The model under review builds one solid part; all positions refer to its coordinate system, in mm. Face numbers are marked on the shaded views. A direction names the side the tool comes from. Coordinates: 2 decimals unless noted, no trailing zeros. Loops run counter-clockwise (first coordinate to the right, second up) from the corner with the lowest first, then second, coordinate; pieces in that order, holes last. Notation, with made-up numbers: (-39, 80) -> (-18, 80) arc R13 cw to (-18, 94) -> close; hole circle Ø5 at (55.5, 72.25). An arc over 180 degrees is marked (long way). One line per question, with ' | ' between items. Start each with the question number.
from build123d import *

# Parameters (mm, degrees)
SKETCH6_W          = 28.575
SKETCH6_H          = 5.588000000000008
FILLET1_R          = 1.524
CUT_EXTRUDE1_DEPTH = 133.3733867563125


with BuildPart() as part:
    # Sweep1: sweep along a path in Sketch1
    with BuildLine(Plane(origin=(0, 0, 0), x_dir=(0, 0, -1), z_dir=(1, 0, 0))) as sweep1_path:
        Line((3.9e-16, 94.996), (0, 0))
        ThreePointArc((0, 0), (37.09799061473534, -40.48535253044856), (80.66258708241622, -7.057061940383765))
        Line((80.66258708241622, -7.057061940383765), (87.31250000000001, 30.656468291151832))
    # Sketch2 → Sweep1 (sweep)
    with BuildSketch(Plane(origin=(0, 94.996, -15.113000000000007), x_dir=(1, 0, 0), z_dir=(0, -1, 0))):
        Polygon((-12.763499999999997, 17.653000000000006), (12.763499999999997, 17.65300000000001), (12.763500000000008, 15.113000000000001), (-12.763499999999983, 15.113000000000001), align=None)
    sweep(path=sweep1_path.line)

    # Sweep3: sweep along a path in Sketch5
    with BuildLine(Plane(origin=(0, 0, 0), x_dir=(0, 0, -1), z_dir=(1, 0, 0))) as sweep3_path:
        Line((0, 63.245999999999995), (-3.47e-15, 3.35e-15))
        ThreePointArc((-3.47e-15, 3.35e-15), (37.09799061473534, -40.48535253044856), (80.66258708241622, -7.057061940383765))
        Line((80.66258708241622, -7.057061940383765), (87.31250000000001, 30.656468291151832))
    # Sketch6 → Sweep3 (sweep)
    with BuildSketch(Plane(origin=(0, 44.66337954391292, -7.875358863214053), x_dir=(1, 0, 0), z_dir=(0, 0.9848077530122094, -0.1736481776669233))):
        with Locations((7.11e-15, 81.9325870824162)):
            Rectangle(SKETCH6_W, SKETCH6_H)
        Polygon((-12.763499999999997, 83.2025870824162), (-12.763499999999983, 80.6625870824162), (12.763500000000008, 80.6625870824162), (12.763499999999997, 83.2025870824162), align=None, mode=Mode.SUBTRACT)
    sweep(path=sweep3_path.line)

    # Fillet1
    fillet1_edges = [part.edges().sort_by_distance(p)[0] for p in [
        (-14.287499999999994, 31.622999999999998, -1.5239999999999834),
        (14.287500000000007, 31.622999999999998, 4.064000000000009),
        (-14.287499999999994, -38.96715181055673, -37.23081596668276),
        (14.287500000000007, -44.53388778349341, -36.74378967620887),
        (14.287500000000009, -38.967151810556715, -37.23081596668276),
        (14.287500000000009, 31.622999999999998, -1.5240000000000133),
        (14.287500000000007, 11.09399698134567, -87.98980224944968),
        (14.287500000000009, 12.06434299814844, -82.48669652561743),
        (-14.287499999999996, -44.53388778349341, -36.74378967620887),
        (-14.287499999999996, 31.622999999999998, 4.064000000000009),
        (-14.287499999999994, 12.06434299814843, -82.48669652561752),
        (-14.287499999999996, 11.09399698134567, -87.98980224944968),
        (14.287500000000007, 30.435935105514844, -88.56320584632552),
        (5.33e-15, 29.950762097113483, -91.31475870824151),
        (-14.287499999999994, 30.435935105514847, -88.56320584632554),
        (7.11e-15, 30.92110811391625, -85.81165298440926),
    ]]
    fillet(fillet1_edges, radius=FILLET1_R)

    # Sketch9 → Cut-Extrude1 (cut, through all)
    with BuildSketch(Plane(origin=(0, 0, 0), x_dir=(-1, 0, 0), z_dir=(0, -6e-17, -1))):
        with BuildLine():
            Line((4.7625, 86.03336979368495), (4.762500000000001, 79.121))
            ThreePointArc((4.762500000000001, 79.121), (-7.9e-16, 68.57086979368498), (-4.762500000000001, 79.121))
            Line((-4.762500000000001, 79.121), (-4.7625, 86.03336979368495))
            ThreePointArc((-4.7625, 86.03336979368495), (1.48e-15, 90.79586979368496), (4.7625, 86.03336979368495))
        make_face()
    extrude(amount=-CUT_EXTRUDE1_DEPTH, mode=Mode.SUBTRACT)


solid = part.part
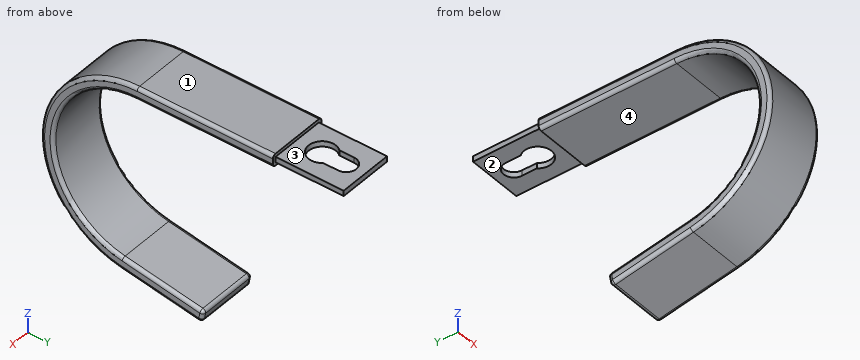
1) Consider section A-A, the plane x = 0. Write out the cut boundary in (y, z), plus the area to 3 significant figures.
2) Consider section B-B, the plane y = 72.5. Write out the cut boundary in (x, z), plus the area to 3 significant figures.
3) Machinability: for the marked faces 1, 2, 3 and 4, which of the approach directions +Z, -Z, +X, -X, +Y, -Y give a long, thin tool a straight path to every point of the face, cutting with its end or side? Answer none if there is none.
4) Consider section C-C, the plane x = 8.5. Write out the cut boundary in (y, z), plus the area to 3 significant figures.
5) Insertion check: pin 1 Ø7.5 at (x, y) = (2, 23) entering from -Z; pin 2 Ø0.8 at (y, z) = (84, 1) entering from -X; pin 3 Ø8 at (x, z) = (5.5, -27) entering from +Y. Each pin has a flat end and moves straight along its axis. Give the tip position at first contact, or say it passes through.
6) Wall thickness on L1, parallel to Z at x = 5.25, y = 69.5; L2, parallel to Z at x = 5.5, y = -26; L3, parallel to Z at x = -12.25, y = 18: over which ranges is each line inside the solid? List them lowest first.
Filled sheet:
1) outline: (-7.76, -84.66) -> (28.45, -91.05) arc R1.52 ccw to (30.22, -89.81) -> (30.66, -87.31) arc R1.52 ccw to (29.42, -85.55) -> (-6.79, -79.16) arc R39.12 cw to (0, -1.52) -> (63.25, -1.52) -> (63.25, 0) -> (68.57, 0) -> (68.57, 2.54) -> (63.25, 2.54) -> (63.25, 4.06) -> (0, 4.06) arc R44.7 ccw to start; (90.8, 0) -> (95, 0) -> (95, 2.54) -> (90.8, 2.54) -> close | area: 1,290 mm^2
2) outline: (-12.76, 0) -> (-5.87, 0) -> (-5.87, 2.54) -> (-12.76, 2.54) -> close; (5.87, 0) -> (12.76, 0) -> (12.76, 2.54) -> (5.87, 2.54) -> close | area: 35.0 mm^2
3) face 1: +Z, +X, -X, +Y, -Y | face 2: -Z, +X, -X, +Y | face 3: +Z, +X, -X, +Y | face 4: +X, -X, +Y
4) outline: (-7.76, -84.66) -> (28.45, -91.05) arc R1.52 ccw to (30.22, -89.81) -> (30.66, -87.31) arc R1.52 ccw to (29.42, -85.55) -> (-6.79, -79.16) arc R39.12 cw to (0, -1.52) -> (63.25, -1.52) -> (63.25, 0) -> (95, 0) -> (95, 2.54) -> (63.25, 2.54) -> (63.25, 4.06) -> (0, 4.06) arc R44.7 ccw to start | area: 1,340 mm^2
5) pin 1: z = -90.75 | pin 2: x = -12.76 | pin 3: y = -34.91
6) L1: 0 to 2.54 | L2: -77.01 to -69.86, -11.42 to -4.27 | L3: -89.21 to -83.53, -1.52 to 4.06
